```python
from build123d import *

# Parameters (mm, degrees)
EXTRUDE_1_DEPTH     = 32
SKETCH_2_W          = 32
SKETCH_2_H          = 12
CUT_EXTRUDE_2_DEPTH = 61.398675482
CUT_EXTRUDE_3_DEPTH = 61.398675482


with BuildPart() as part:
    # 草圖1 → 伸長1 (new, symmetric)
    with BuildSketch(Plane(origin=(0, 0, 0), x_dir=(0, 0, -1), z_dir=(1, 0, 0))):
        Polygon((0, 0), (0, 10), (30, 32), (40, 32), (40, 0), align=None)
    extrude(amount=EXTRUDE_1_DEPTH, both=True)

    # 草圖2 → 伸長2 (cut, through all)
    with BuildSketch(Plane(origin=(0, 0, 0), x_dir=(-1, 0, 0), z_dir=(0, 0, -1))):
        with Locations((0, 26)):
            Rectangle(SKETCH_2_W, SKETCH_2_H)
    extrude(amount=CUT_EXTRUDE_2_DEPTH, mode=Mode.SUBTRACT)

    # 草圖3 → 伸長3 (cut, through all)
    with BuildSketch(Plane.XZ):
        Polygon((-32, -10), (-32, 0), (-20, 0), align=None)
        Polygon((32, -10), (32, 0), (20, 0), align=None)
    extrude(amount=-CUT_EXTRUDE_3_DEPTH, mode=Mode.SUBTRACT)


solid = part.part
```
Check sheet for the modelled part. Datum: model origin and axes. Units: mm. A direction names the side the tool comes from. Round coordinates to 2 decimals unless told otherwise and drop trailing zeros. Loops run counter-clockwise (first coordinate to the right, second up) from the corner with the lowest first, then second, coordinate; pieces in that order, holes last. Notation, with made-up numbers: (64.5, 17.25) - (107.5, 17.25) arc R18 cw to (107.5, 33.25) - close; hole circle Ø1 at (68, 48). An arc over 180 degrees is marked (long way). Answer as a JSON object with one key per item and string values. Group by question number.
Q1. Sectioned sample at B-B, the plane y = 6. Enter the section's corners in (x, z), plus the area to 3 significant figures.
Q2. Sectioned sample at D-D, the plane y = 22. Enter the section's corners in (x, z), plus the area to 3 significant figures.
Q3. Sectioned sample at A-A, the plane z = -31. Enter the section's corners in (x, y).
Q4. Set-up check for faces 1 (the face through (-24, 32, -35)), 2 (the face through (16, 25, -30)): record each of +Z, -Z, +X, -X, +Y, -Y from which the full face is reachable in a straight line by a thin tool's end or side.
Q5. Mould release check, pull along X, two halves, no side actions. Record for faces 3 (the face through (-16, 25, -30)), 4 (the face through (0, 5, 0)), 5 (the face through (-26, 7, -5)): released by +X, released by -X, zero draft, split by the parting line, or undercut.
Q6. Scan lines: line 1 along X through (y, z) = (23, -21); line 2 along Y through (x, z) = (-10, -19); line 3 along Z through (x, y) = (-18, 20.5). Record each from-to range of solid material in increasing order. Write a range as [from, to].
Q7. Gauge pin test, flat ends, axial feed: P1, Ø12, axis at x = 17, y = 15, coming from the +Z side; P2, Ø6, axis at x = 23.5, z = -19.5, coming from the +Y side; P3, Ø4, axis at x = 5, y = 18.5, coming from the +Z side; P4, Ø1.5, axis at x = 22, z = -12.5, coming from the +Y side. Record the tip position at first contact, or that the pin passes through.
Q8. Sectioned sample at C-C, the plane x = -4.5. Enter the section's corners in (y, z).
Solution:
{
 "1": {"outline": "(-32, -40) - (32, -40) - (32, -10) - (20, 0) - (-20, 0) - (-32, -10) - close", "area": "2,440 mm²"},
 "2": {"outline": "(-32, -40) - (-16, -40) - (-16, -16.36) - (-32, -16.36) - close; (16, -40) - (32, -40) - (32, -16.36) - (16, -16.36) - close", "area": "756 mm²"},
 "3": {"outline": "(-32, 0) - (32, 0) - (32, 32) - (16, 32) - (16, 20) - (-16, 20) - (-16, 32) - (-32, 32) - close"},
 "4": {"face 1": "+Z, -Z, +X, -X, +Y", "face 2": "+Z, -Z, +Y"},
 "5": {"face 3": "undercut", "face 4": "zero draft", "face 5": "released by -X"},
 "6": {"line 1": "x = [-32, -16], [16, 32]", "line 2": "y = [0, 20]", "line 3": "z = [-40, -14.32]"},
 "7": {"P1": "stops at z = 0", "P2": "stops at y = 26.5", "P3": "stops at z = -8.86", "P4": "stops at y = 19.72"},
 "8": {"outline": "(0, -40) - (20, -40) - (20, -13.64) - (10, 0) - (0, 0) - close"}
}
